```python
from build123d import *

# Parameters (mm, degrees)
SKETCH1_W           = 30
SKETCH1_H           = 8
BOSS_EXTRUDE1_DEPTH = 3
SKETCH2_R           = 1.5
CUT_EXTRUDE1_DEPTH  = 4
FILLET1_R           = 3.5
SCALE1_SCALE        = 0.75
SCALE2_SCALE        = 0.7


with BuildPart() as part:
    # Sketch1 → Boss-Extrude1 (new body)
    with BuildSketch(Plane(origin=(0, 0, 0), x_dir=(0, 1, 0), z_dir=(0, 0, 1))):
        Rectangle(SKETCH1_W, SKETCH1_H)
    extrude(amount=-BOSS_EXTRUDE1_DEPTH)

    # Sketch2 → Cut-Extrude1 (cut)
    with BuildSketch(Plane.XY):
        with Locations((0, 11)):
            Circle(SKETCH2_R)
        with Locations((0, -11)):
            Circle(SKETCH2_R)
    extrude(amount=-CUT_EXTRUDE1_DEPTH, mode=Mode.SUBTRACT)

    # Fillet1
    fillet1_edges = [part.edges().sort_by_distance(p)[0] for p in [
        (4, 15, -1.5),
        (4, -15, -1.5),
        (-4, -15, -1.5),
        (-4, 15, -1.5),
    ]]
    fillet(fillet1_edges, radius=FILLET1_R)


with BuildPart() as part_1:
    # Scale1: scaled about (0, 0, -1.5)
    add(part.part.scale(SCALE1_SCALE).moved(Location((0, 0, -0.375))))


with BuildPart() as part_2:
    # Scale2: scaled about (0, 0, -1.5)
    add(part_1.part.scale(SCALE2_SCALE).moved(Location((0, 0, -0.45))))


solid = part_2.part
```
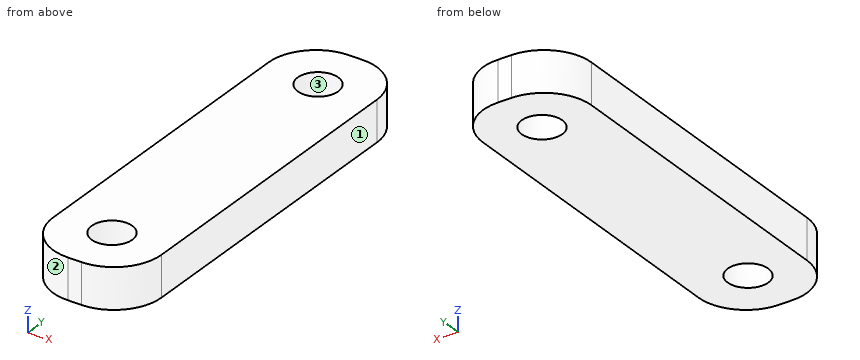
Could you check a few things on this model? Use its own coordinates, in mm. Face numbers are marked on the shaded views. Round coordinates to 2 decimals unless told otherwise and drop trailing zeros. Loops run counter-clockwise (first coordinate to the right, second up) from the corner with the lowest first, then second, coordinate; pieces in that order, holes last.
Q1. I want a section at C-C (x = -1.55). Write out the boundary of the cut face in (y, z), and give its area (3 significant figures).
Q2. Please list where these lines run through material, in increasing order: L1, parallel to Y at x = 0, z = -1.8 (1 decimal); L2, parallel to Y at x = 0.65, z = -1.95; L3, parallel to X at y = 6, z = -1.
Q3. I want a section at B-B (z = -1.4). Write out the boundary of the cut face in (x, y) (1 decimal), and give its area (3 significant figures).
Q4. I want a section at D-D (x = 0.95). Write out the boundary of the cut face in (y, z), and give its area (3 significant figures).
Q5. For P1, Ø1.3, axis at x = 0, y = 5.775, coming from the -Z side; P2, Ø2, axis at x = -0.5, y = -5.5, coming from the -Z side, each with a flat end and sliding along its axis, tell me the tip position at first contact or that it passes through.
Q6. Thinking about a two-plate mould opening in X: for the marked faces 1, 2 and 3, which applies, pulls with the +X half, pulls with the -X half, needs draft (parallel to the pull), parting line crosses it, or undercut?
Q7. I want a section at A-A (x = 0). Write out the boundary of the cut face in (y, z) (1 decimal).
Answer below:
1. outline: (-7.35, -2.29) - (7.35, -2.29) - (7.35, -0.71) - (-7.35, -0.71) - close
1. area: 23.1 mm2
2. L1: y = -7.9 to -6.6, -5 to 5, 6.6 to 7.9
2. L2: y = -7.83 to -6.22, -5.33 to 5.33, 6.22 to 7.83
2. L3: x = -2.1 to -0.75, 0.75 to 2.1
3. outline: (-2.1, -6) arc R1.8 ccw to (-0.3, -7.9) - (0.3, -7.9) arc R1.8 ccw to (2.1, -6) - (2.1, 6) arc R1.8 ccw to (0.3, 7.9) - (-0.3, 7.9) arc R1.8 ccw to (-2.1, 6) - close; hole circle Ø1.6 at (0, -5.8); hole circle Ø1.6 at (0, 5.8)
3. area: 59.4 mm2
4. outline: (-7.74, -2.29) - (7.74, -2.29) - (7.74, -0.71) - (-7.74, -0.71) - close
4. area: 24.4 mm2
5. P1: passes through
5. P2: stops at z = -2.29
6. face 1: pulls with the +X half
6. face 2: pulls with the -X half
6. face 3: undercut
7. outline: (-7.9, -2.3) - (-6.6, -2.3) - (-6.6, -0.7) - (-7.9, -0.7) - close; (-5, -2.3) - (5, -2.3) - (5, -0.7) - (-5, -0.7) - close; (6.6, -2.3) - (7.9, -2.3) - (7.9, -0.7) - (6.6, -0.7) - close
